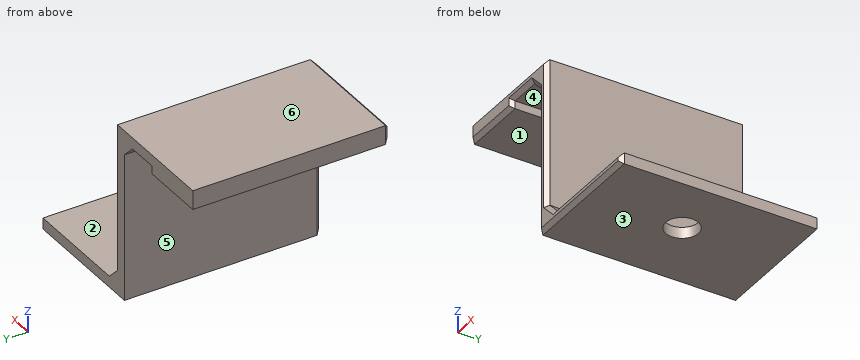
```python
from build123d import *

# Parameters (mm, degrees)
F1_DEPTH = 30
F2_SIZE  = 2
F3_SIZE  = 0.6
F4_R     = 2.5
F5_DEPTH = 1.7


with BuildPart() as f1:
    # F0 (on Front) → F1 (new body)
    with BuildSketch(Plane.XZ):
        Polygon((0, 24.5), (0, 0), (20, 0), (20, 1.7), (1.7, 1.7), (1.7, 26.2), (-16.8, 26.2), (-16.8, 23.3), (-6.8, 23.3), (-6.8, 24.5), align=None)
    extrude(amount=-F1_DEPTH)

    # F2
    f2_edges = [f1.edges().sort_by_distance(p)[0] for p in [
        (1.7, 15, 1.7),
        (0, 15, 24.5),
    ]]
    chamfer(f2_edges, length=F2_SIZE)

    # F3
    f3_edges = [f1.edges().sort_by_distance(p)[0] for p in [
        (1.7, 0, 14.95),
        (2.7, 0, 2.7),
        (-7.55, 0, 26.2),
        (11.85, 0, 1.7),
        (-16.8, 0, 24.75),
        (20, 0, 0.85),
        (-11.8, 0, 23.3),
        (10, 0, 0),
        (-6.8, 0, 23.9),
        (0, 0, 11.25),
        (-4.4, 0, 24.5),
        (-1, 0, 23.5),
    ]]
    chamfer(f3_edges, length=F3_SIZE)

    # F4 (on face) → F5 (cut, through all)
    with BuildSketch(Plane(origin=(0, 0, 0), x_dir=(1, 0, 0), z_dir=(0, 0, -1))):
        with Locations((11, -15)):
            Circle(F4_R)
    extrude(amount=-F5_DEPTH, mode=Mode.SUBTRACT)


solid = f1.part
```
Work out the finished part from the listing and answer in its coordinate system (mm). Face numbers are marked on the shaded views. A direction names the side the tool comes from. Round coordinates to 2 decimals unless told otherwise and drop trailing zeros. Write each loop counter-clockwise with the first axis right and the second up, starting at its lowest first coordinate (ties: lowest second). Pieces come first, ordered by that corner, then holes.
1) A cutting plane is placed at C-C on y = 22.5. Determine the outline of the cut face in (x, z), and give its area (3 significant figures).
2) A cutting plane is placed at D-D on z = 19.5. Determine the outline of the cut face in (x, y).
3) Consider probe 1 along X at (y, z) = (15, 1.35); probe 2 along Y at (x, z) = (11, 0.7); probe 3 along Z at (x, y) = (4.5, 18.5). Determine where each line is inside the solid, lowest interval first.
4) A cutting plane is placed at B-B on x = 11. Determine the outline of the cut face in (y, z).
5) Determine the mould class of the marked faces 4, 5 and 6 for opening direction X: pulls with the +X half, pulls with the -X half, needs draft (parallel to the pull), parting line crosses it, or undercut.
6) Flat-ended cylindrical pins translate along their axes: P1, Ø10, axis at y = 10, z = 17.5, coming from the +X side; P2, Ø6, axis at y = 12.5, z = 15.5, coming from the -X side; P3, Ø5, axis at x = -13, y = 18.5, coming from the -Z side. Find the tip coordinate at first contact, or state that the pin passes through.
7) A cutting plane is placed at A-A on y = 15. Determine the outline of the cut face in (x, z), and give its area (3 significant figures).
8) Which of the six approach directions +Z, -Z, +X, -X, +Y, -Y give full straight-line access (tool end or side, diameter ignored) to the marked faces 1, 2 and 3?
Entries:
1. outline: (-16.8, 23.3) - (-6.8, 23.3) - (-6.8, 24.5) - (-2, 24.5) - (0, 22.5) - (0, 0) - (20, 0) - (20, 1.7) - (3.7, 1.7) - (1.7, 3.7) - (1.7, 26.2) - (-16.8, 26.2) - close
1. area: 120 mm2
2. outline: (0, 0.6) - (0.6, 0) - (1.1, 0) - (1.7, 0.6) - (1.7, 30) - (0, 30) - close
3. probe 1: x = 0 to 8.5, 13.5 to 20
3. probe 2: y = 0 to 12.5, 17.5 to 30
3. probe 3: z = 0 to 1.7
4. outline: (0, 0.6) - (0.6, 0) - (12.5, 0) - (12.5, 1.7) - (0.6, 1.7) - (0, 1.1) - close; (17.5, 0) - (30, 0) - (30, 1.7) - (17.5, 1.7) - close
5. face 4: undercut
5. face 5: pulls with the -X half
5. face 6: needs draft
6. P1: stops at x = 1.7
6. P2: stops at x = 0
6. P3: stops at z = 23.3
7. outline: (-16.8, 23.3) - (-6.8, 23.3) - (-6.8, 24.5) - (-2, 24.5) - (0, 22.5) - (0, 0) - (8.5, 0) - (8.5, 1.7) - (3.7, 1.7) - (1.7, 3.7) - (1.7, 26.2) - (-16.8, 26.2) - close; (13.5, 0) - (20, 0) - (20, 1.7) - (13.5, 1.7) - close
7. area: 112 mm2
8. face 1: -Z, -X, +Y, -Y
8. face 2: +Z, +X, +Y, -Y
8. face 3: -Z, +X, -X, +Y, -Y
